```python
from build123d import *

# Parameters (mm, degrees)
F0_W     = 5
F0_H     = 20
F0_R     = 2.25
F0_W_2   = 16.5
F0_H_2   = 5
F1_DEPTH = 8
F2_R     = 3.99999
F4_DEPTH = 5


# Not quite as in the source:
# - a fillet or chamfer is up to 0.001 mm smaller than in the source, because OpenCascade refuses the exact size
# - a feature names something its author has since deleted; it is built from what else it names


with BuildPart() as f1:
    # F0 (on Top) → F1 (new body)
    with BuildSketch(Plane.XY):
        Rectangle(F0_W, F0_H)
        Polygon((-2.5, 10), (2.5, 10), (3.5, 10), (3.5, 17), (-3.5, 17), (-3.5, 16), (-3.5, 11), (-3.5, 10), align=None)
        with Locations((0, 13.5)):
            Circle(F0_R, mode=Mode.SUBTRACT)
        with Locations((-11.75, 13.5)):
            Rectangle(F0_W_2, F0_H_2)
    extrude(amount=F1_DEPTH)

    # F2 (radius 4 in the source; OpenCascade refuses exactly that, so slightly less here)
    f2_edges = [f1.edges().sort_by_distance(p)[0] for p in [
        (-2.5, 0, 8),
        (-2.5, 0, 0),
    ]]
    fillet(f2_edges, radius=F2_R)

    # F3 (on face) → F4 (cut)
    with BuildSketch(Plane.XY.offset(8)):
        with BuildLine():
            ThreePointArc((-15.8291561976, 16), (-15, 16.25), (-14.1708438024, 16))
            Line((-14.1708438024, 16), (-12.8349364905, 16))
            ThreePointArc((-12.8349364905, 16), (-15, 17.25), (-17.1650635095, 16))
            Line((-17.1650635095, 16), (-15.8291561976, 16))
        make_face()
        with BuildLine():
            ThreePointArc((-14.1708438024, 16), (-13.6783089816, 15.4593185827), (-13.5, 14.75))
            ThreePointArc((-13.5, 14.75), (-15.7093185827, 13.4283089816), (-15.8291561976, 16))
            Line((-15.8291561976, 16), (-17.1650635095, 16))
            ThreePointArc((-17.1650635095, 16), (-15.6470476128, 12.3351854343), (-12.5, 14.75))
            ThreePointArc((-12.5, 14.75), (-12.5851854343, 15.3970476128), (-12.8349364905, 16))
            Line((-12.8349364905, 16), (-14.1708438024, 16))
        make_face()
    extrude(amount=-F4_DEPTH, mode=Mode.SUBTRACT)


solid = f1.part
```
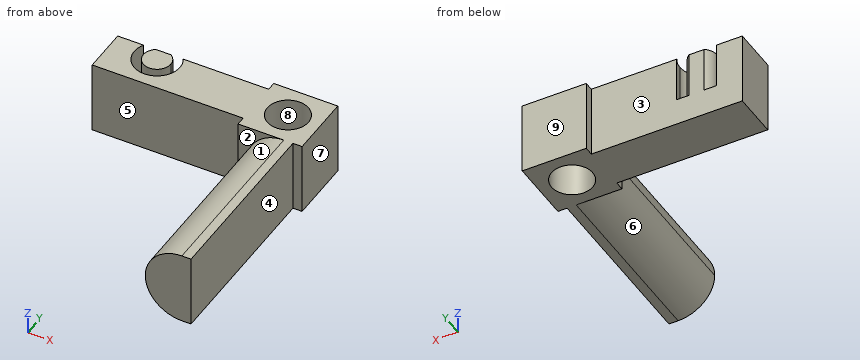
Verification items for the finished model (mm, model axes). Face numbers are marked on the shaded views. A direction names the side the tool comes from. Give positions to 0.01 mm unless a question says otherwise; leave off trailing zeros. Order: outer loops, then holes, each group sorted by start corner. A loop starts at its lowest first (then second) coordinate and runs counter-clockwise, first axis right, second up. Notation, with made-up numbers: M 32.25,33.5 L 41.25,33.5 A37 ccw 41.25,70.5 Z; hole C 2.25,48 d4. An arc over 180 degrees is marked long. Answer in a Markdown table with one row per item. Add a question column.
Item 1: Gauge pin test, flat ends, axial feed: pin 1 (0.8 mm diameter, centred on y = 16.5, z = 6, fed in from -X); pin 2 (2.5 mm diameter, centred on y = 3, z = 5, fed in from +X); pin 3 (2.5 mm diameter, centred on x = -13.5, z = 3.5, fed in from -Y). Record the tip position at first contact, or that the pin passes through.
Item 2: Scan lines: probe 1 along Y at (x, z) = (-15, 5.2); probe 2 along Y at (x, z) = (0, 1.75); probe 3 along X at (y, z) = (14.75, 5.4). Record each from-to range of solid material in increasing order. Write a range as from..to.
Item 3: Tool access check on the marked faces 1, 2, 3, 4 and 5. Record the directions out of +Z, -Z, +X, -X, +Y, -Y that give a thin tool (end or side, any length) a straight path to the whole face; none if there is none.
Item 4: Mould release check, pull along X, two halves, no side actions. Record for the marked faces 6, 7, 8 and 9: released by +X, released by -X, zero draft, split by the parting line, or undercut.
Item 5: Section check A-A, the plane z = 5.5. Enter the section's corners in (x, y), and give its area (3 significant figures).
Item 6: Section check B-B, the plane x = 0. Enter the section's corners in (y, z).
Item 7: Section check C-C, the plane z = 2.25. Enter the section's corners in (x, y), and give its area (3 significant figures).
Filled sheet:
| question | item | result |
|---|---|---|
| 1 | pin 1 | stops at x = -3.5 |
| 1 | pin 2 | stops at x = 2.5 |
| 1 | pin 3 | stops at y = 11 |
| 2 | probe 1 | y = 11..12.25, 13.25..16 |
| 2 | probe 2 | y = -10..11.25, 15.75..17 |
| 2 | probe 3 | x = -20..-17.5, -16.5..-13.5, -12.5..-1.87, 1.87..3.5 |
| 3 | face 1 | +Z, -X, -Y |
| 3 | face 2 | +Z, -X, -Y |
| 3 | face 3 | +Z, -Z, -X, +Y |
| 3 | face 4 | +Z, -Z, +X, -Y |
| 3 | face 5 | +Z, -Z, -X, -Y |
| 4 | face 6 | released by -X |
| 4 | face 7 | released by +X |
| 4 | face 8 | undercut |
| 4 | face 9 | zero draft |
| 5 | outline | M -20,11 L -3.5,11 L -3.5,10 L -2.21,10 L -2.21,-10 L 2.5,-10 L 2.5,10 L 3.5,10 L 3.5,17 L -3.5,17 L -3.5,16 L -12.83,16 A2.5 cw long -17.17,16 L -20,16 Z; M -15.83,16 A1.5 ccw long -14.17,16 Z; hole C 0,13.5 d4.5 |
| 5 | area | 201 mm^2 |
| 6 | outline | M -10,0.29 L 10,0.29 L 10,0 L 11.25,0 L 11.25,8 L 10,8 L 10,7.71 L -10,7.71 Z; M 15.75,0 L 17,0 L 17,8 L 15.75,8 Z |
| 7 | outline | M -20,11 L -3.5,11 L -3.5,10 L -2.1,10 L -2.1,-10 L 2.5,-10 L 2.5,10 L 3.5,10 L 3.5,17 L -3.5,17 L -3.5,16 L -20,16 Z; hole C 0,13.5 d4.5 |
| 7 | area | 208 mm^2 |
